from build123d import *

# Parameters (mm, degrees)
CROQUIS1_R              = 5.85
SALIENTE_EXTRUIR1_DEPTH = 480


with BuildPart() as part:
    # Croquis1 → Saliente-Extruir1 (new body)
    with BuildSketch(Plane.XY):
        with BuildLine():
            Line((-17.5, -5), (-16, -5))
            ThreePointArc((-16, -5), (-15.646446609, -5.146446609), (-15.5, -5.5))
            Line((-15.5, -5.5), (-15.5, -9.5))
            ThreePointArc((-15.5, -9.5), (-15.353553391, -9.853553391), (-15, -10))
            Line((-15, -10), (-11.790147321, -10))
            ThreePointArc((-11.790147321, -10), (-11.539192936, -9.932460283), (-11.356036103, -9.748087586))
            Line((-11.356036103, -9.748087586), (-9.065888782, -5.740718013))
            ThreePointArc((-9.065888782, -5.740718013), (-9.016752854, -5.620974478), (-9, -5.492630427))
            Line((-9, -5.492630427), (-9, 5.492630427))
            ThreePointArc((-9, 5.492630427), (-9.016752854, 5.620974478), (-9.065888782, 5.740718013))
            Line((-9.065888782, 5.740718013), (-11.356036103, 9.748087586))
            ThreePointArc((-11.356036103, 9.748087586), (-11.539192936, 9.932460283), (-11.790147321, 10))
            Line((-11.790147321, 10), (-15, 10))
            ThreePointArc((-15, 10), (-15.353553391, 9.853553391), (-15.5, 9.5))
            Line((-15.5, 9.5), (-15.5, 5.5))
            ThreePointArc((-15.5, 5.5), (-15.646446609, 5.146446609), (-16, 5))
            Line((-16, 5), (-17.5, 5))
            Line((-17.5, 5), (-17.5, 14))
            ThreePointArc((-17.5, 14), (-16.474873734, 16.474873734), (-14, 17.5))
            Line((-14, 17.5), (-5, 17.5))
            Line((-5, 17.5), (-5, 16))
            ThreePointArc((-5, 16), (-5.146446609, 15.646446609), (-5.5, 15.5))
            Line((-5.5, 15.5), (-9.5, 15.5))
            ThreePointArc((-9.5, 15.5), (-9.853553391, 15.353553391), (-10, 15))
            Line((-10, 15), (-10, 11.790147321))
            ThreePointArc((-10, 11.790147321), (-9.932460283, 11.539192936), (-9.748087586, 11.356036103))
            Line((-9.748087586, 11.356036103), (-5.740718013, 9.065888782))
            ThreePointArc((-5.740718013, 9.065888782), (-5.620974478, 9.016752854), (-5.492630427, 9))
            Line((-5.492630427, 9), (5.492630427, 9))
            ThreePointArc((5.492630427, 9), (5.620974478, 9.016752854), (5.740718013, 9.065888782))
            Line((5.740718013, 9.065888782), (9.748087586, 11.356036103))
            ThreePointArc((9.748087586, 11.356036103), (9.932460283, 11.539192936), (10, 11.790147321))
            Line((10, 11.790147321), (10, 15))
            ThreePointArc((10, 15), (9.853553391, 15.353553391), (9.5, 15.5))
            Line((9.5, 15.5), (5.5, 15.5))
            ThreePointArc((5.5, 15.5), (5.146446609, 15.646446609), (5, 16))
            Line((5, 16), (5, 17.5))
            Line((5, 17.5), (14, 17.5))
            ThreePointArc((14, 17.5), (16.474873734, 16.474873734), (17.5, 14))
            Line((17.5, 14), (17.5, 5))
            Line((17.5, 5), (16, 5))
            ThreePointArc((16, 5), (15.646446609, 5.146446609), (15.5, 5.5))
            Line((15.5, 5.5), (15.5, 9.5))
            ThreePointArc((15.5, 9.5), (15.353553391, 9.853553391), (15, 10))
            Line((15, 10), (11.790147321, 10))
            ThreePointArc((11.790147321, 10), (11.539192936, 9.932460283), (11.356036103, 9.748087586))
            Line((11.356036103, 9.748087586), (9.065888782, 5.740718013))
            ThreePointArc((9.065888782, 5.740718013), (9.016752854, 5.620974478), (9, 5.492630427))
            Line((9, 5.492630427), (9, -5.492630427))
            ThreePointArc((9, -5.492630427), (9.016752854, -5.620974478), (9.065888782, -5.740718013))
            Line((9.065888782, -5.740718013), (11.356036103, -9.748087586))
            ThreePointArc((11.356036103, -9.748087586), (11.539192936, -9.932460283), (11.790147321, -10))
            Line((11.790147321, -10), (15, -10))
            ThreePointArc((15, -10), (15.353553391, -9.853553391), (15.5, -9.5))
            Line((15.5, -9.5), (15.5, -5.5))
            ThreePointArc((15.5, -5.5), (15.646446609, -5.146446609), (16, -5))
            Line((16, -5), (17.5, -5))
            Line((17.5, -5), (17.5, -14))
            ThreePointArc((17.5, -14), (16.474873734, -16.474873734), (14, -17.5))
            Line((14, -17.5), (5, -17.5))
            Line((5, -17.5), (5, -16))
            ThreePointArc((5, -16), (5.146446609, -15.646446609), (5.5, -15.5))
            Line((5.5, -15.5), (9.5, -15.5))
            ThreePointArc((9.5, -15.5), (9.853553391, -15.353553391), (10, -15))
            Line((10, -15), (10, -11.790147321))
            ThreePointArc((10, -11.790147321), (9.932460283, -11.539192936), (9.748087586, -11.356036103))
            Line((9.748087586, -11.356036103), (5.740718013, -9.065888782))
            ThreePointArc((5.740718013, -9.065888782), (5.620974478, -9.016752854), (5.492630427, -9))
            Line((5.492630427, -9), (-5.492630427, -9))
            ThreePointArc((-5.492630427, -9), (-5.620974478, -9.016752854), (-5.740718013, -9.065888782))
            Line((-5.740718013, -9.065888782), (-9.748087586, -11.356036103))
            ThreePointArc((-9.748087586, -11.356036103), (-9.932460283, -11.539192936), (-10, -11.790147321))
            Line((-10, -11.790147321), (-10, -15))
            ThreePointArc((-10, -15), (-9.853553391, -15.353553391), (-9.5, -15.5))
            Line((-9.5, -15.5), (-5.5, -15.5))
            ThreePointArc((-5.5, -15.5), (-5.146446609, -15.646446609), (-5, -16))
            Line((-5, -16), (-5, -17.5))
            Line((-5, -17.5), (-14, -17.5))
            ThreePointArc((-14, -17.5), (-16.474873734, -16.474873734), (-17.5, -14))
            Line((-17.5, -14), (-17.5, -5))
        make_face()
        Circle(CROQUIS1_R, mode=Mode.SUBTRACT)
    extrude(amount=SALIENTE_EXTRUIR1_DEPTH)


solid = part.part
Input: part model. Units: mm. Frame: model coordinates. Give positions to 0.01 mm unless a question says otherwise; leave off trailing zeros. Write each loop counter-clockwise with the first axis right and the second up, starting at its lowest first coordinate (ties: lowest second). Pieces come first, ordered by that corner, then holes. Notation, with made-up numbers: M -20,-10 L 12,-10 A16 cw 12,11 Z; hole C 3,0 d8. An arc over 180 degrees is marked long. Use one line per item in the form item = value.
1. Cut plane A-A on y = 0. Return loops of the section in (x, z), and give its area (3 significant figures).
Outcome:
outline = M -9,0 L -5.85,0 L -5.85,480 L -9,480 Z; M 5.85,0 L 9,0 L 9,480 L 5.85,480 Z
area = 3,020 mm²
2. Mould query, pull axis Y, two halves, no side actions, for faces 1 (the face through (10, -17.5, 237)), 2 (the face through (17.5, -9, 237)), 3 (the face through (-9, 0, 237)). Classes: released by +Y, released by -Y, zero draft, split by the parting line, or undercut.
Outcome:
face_1 = released by -Y
face_2 = zero draft
face_3 = undercut
3. First-contact query: P1, Ø12, axis at y = 2, z = 357.5, coming from the -X side; P2, Ø1.2, axis at y = -17, z = 335, coming from the -X side; P3, Ø1.2, axis at y = -16.5, z = 295, coming from the +X side. Flat tips, straight axial feed; report the tip coordinate or a pass-through.
Outcome:
P1 = -17.5
P2 = -16.55
P3 = 16.94
4. Ray query, L1, parallel to Y at x = 7, z = 20; L2, parallel to X at y = 12, z = 360; L3, parallel to Y at x = -3, z = 171. Return the intervals inside material, ascending.
Outcome:
L1 = -17.5 to -15.5, -9.79 to 9.79, 15.5 to 17.5
L2 = -17.5 to -10, 10 to 17.5
L3 = -9 to -5.02, 5.02 to 9
